Autodesk Inventor part; units mm, degrees
ref_plane "YZ Plane" through (0, 0, 0) normal (1, 0, 0) x (0, 1, 0)
ref_plane "XZ Plane" through (0, 0, 0) normal (0, 1, 0) x (-1, 0, 0)
ref_plane "XY Plane" through (0, 0, 0) normal (0, 0, 1) x (1, 0, 0)
sketch "Sketch1" plane through (0, 0, 0) normal (0, 1, 0) x (-1, 0, 0)
  circle A0 centre (0, 0) radius 22.479
  circle A1 centre (0, 0) radius 25.654
  dimension "d0" = 44.958
  dimension "d1" = 51.308
extrude "Extrusion1" add sketch "Sketch1" against normal blind 101.6
sketch "Sketch7" plane through (0, -101.6, 0) normal (0, -1, 0) x (1, 0, 0)
  line L0 (0, 0) -> (25.654, 0) construction
  circle A0 centre (0, 0) radius 25.654 construction
  line L1 (19.304, 3.429) -> (19.304, -3.429)
  line L2 (19.304, -3.429) -> (25.654, -3.429)
  line L3 (25.654, -3.429) -> (25.654, 3.429)
  line L4 (25.654, 3.429) -> (19.304, 3.429)
  circle A1 centre (0, 0) radius 22.479
  line L5 (19.304, 3.429) -> (25.654, -3.429) construction
  line L6 (19.304, -3.429) -> (25.654, 3.429) construction
  point P0 (20.2202, 0)
  point P1 (22.479, 0)
  dimension "d10" = 6.858
  dimension "d11" = 6.35
extrude "Extrusion2" cut sketch "Sketch7" against normal blind 101.6 contours L4 A1 L2 L1 | L4 L3 L2 A1 picked at (20.3623, 0)
sketch "Sketch8" plane through (0, -101.6, 0) normal (0, -1, 0) x (1, 0, 0)
  circle A0 centre (0, 0) radius 25.654
  circle A1 centre (0, 0) radius 38.1
  dimension "d14" = 51.308
  dimension "d15" = 76.2
extrude "Extrusion3" add sketch "Sketch8" against normal blind 12.7
sketch "Sketch10" plane through (0, -101.6, 0) normal (0, -1, 0) x (1, 0, 0)
  circle A0 centre (31.75, 0) radius 2.4257
  circle A1 centre (15.875, 27.4963) radius 2.4257
  circle A2 centre (-15.875, 27.4963) radius 2.4257
  circle A3 centre (-31.75, 0) radius 2.4257
  circle A4 centre (-15.875, -27.4963) radius 2.4257
  circle A5 centre (15.875, -27.4963) radius 2.4257
  point P0 (0, 0)
  dimension "d30" = 4.8514
  dimension "d33" = 360
extrude "Extrusion4" cut sketch "Sketch10" against normal blind 7.1374
sketch "Sketch11" plane through (31.75, -94.4626, 0) normal (0, -1, 0) x (1, 0, 0)
  point P0 (-31.75, 0)
  point P1 (0, 0)
  point P2 (-15.875, 27.4963)
  point P3 (-47.625, 27.4963)
  point P4 (-63.5, 0)
  point P5 (-47.625, -27.4963)
  point P6 (-15.875, -27.4963)
  dimension "d39" = 360
hole "Hole2" at (31.75, -94.4626, 0) at (15.875, -94.4626, 27.4963) at (-15.875, -94.4626, 27.4963) at (-31.75, -94.4626, 0) at (-15.875, -94.4626, -27.4963) at (15.875, -94.4626, -27.4963) direction (0, 1, 0) diameter 3.81 end through all
properties part number "ExternalStationaryOuterRingOld" material "LCP Plastic"
Verification items for the finished model (mm, model axes). A direction names the side the tool comes from. Round coordinates to 2 decimals unless told otherwise and drop trailing zeros. Order: outer loops, then holes, each group sorted by start corner. A loop starts at its lowest first (then second) coordinate and runs counter-clockwise, first axis right, second up.
1. Section check B-B on z = -17.5. Record the cut outline in (x, y).
Final values:
outline: (-33.84, -101.6) - (-14.11, -101.6) - (-14.11, 0) - (-18.76, 0) - (-18.76, -88.9) - (-33.84, -88.9) - close; (14.11, -101.6) - (33.84, -101.6) - (33.84, -88.9) - (18.76, -88.9) - (18.76, 0) - (14.11, 0) - close
2. Release check for a two-part mould opening along X. For faces 4 (the flat face through (-15, 0, 17)), 5 (the cylindrical face through (25.654, -95.339, -0.048)) record: +X half, -X half, draft (parallel to the pull), parting line (faces both ways), or undercut.
Final values:
face 4: draft
face 5: undercut
3. Section check A-A on x = 0. Record the cut outline in (y, z), then the cut area to 3 significant figures.
Final values:
outline: (-101.6, -38.1) - (-88.9, -38.1) - (-88.9, -25.65) - (0, -25.65) - (0, -22.48) - (-101.6, -22.48) - close; (-101.6, 22.48) - (0, 22.48) - (0, 25.65) - (-88.9, 25.65) - (-88.9, 38.1) - (-101.6, 38.1) - close
area: 961 mm2
4. Go/stop test with flat-tipped pins: P1, Ø8, axis at x = -3.5, y = -72, coming from the -Z side; P2, Ø1, axis at x = 24, y = -26, coming from the -Z side; P3, Ø1.6, axis at x = 24.5, y = -67.5, coming from the +Z side. Record where each tip stops, or that it passes through.
Final values:
P1: stops at z = -25.65
P2: stops at z = -10.29
P3: stops at z = 9.82
5. Section check C-C on y = -10. Record the cut outline in (x, z).
Final values:
outline: (22.22, -3.43) arc R22.48 cw (long way) to (22.22, 3.43) - (25.42, 3.43) arc R25.65 ccw (long way) to (25.42, -3.43) - close
6. Access from +Z, -Z, +X, -X, +Y, -Y to the whole of each face (thin tool, end or side, straight path). Record for faces 1 (the cylindrical face through (-29.89, -91.64, 0.41)), 2 (the flat face through (-18, -94.463, -28)), 3 (the flat face through (-9, -88.9, -25)).
Final values:
face 1: +Y, -Y
face 2: -Y
face 3: +Y
7. Thickness scan on L1, parallel to Z at x = -16, y = -89.5; L2, parallel to X at y = -12, z = 18; L3, parallel to Y at x = -27.5, z = -26. Record the ranges inside material, lowest first.
Final values:
L1: z = -34.58 to -29.4, -25.6 to -15.79, 15.79 to 25.6, 29.4 to 34.58
L2: x = -18.28 to -13.46, 13.46 to 18.28
L3: y = -101.6 to -88.9
